Autodesk Inventor part; units mm, degrees
ref_plane "YZ Plane" through (0, 0, 0) normal (1, 0, 0) x (0, 1, 0)
ref_plane "XZ Plane" through (0, 0, 0) normal (0, 1, 0) x (-1, 0, 0)
ref_plane "XY Plane" through (0, 0, 0) normal (0, 0, 1) x (1, 0, 0)
sketch "スケッチ1" plane through (0, 0, 0) normal (0, 0, 1) x (1, 0, 0)
  line L0 (0, 0) -> (10, 0)
  line L1 (10, 0) -> (10, 30)
  line L2 (10, 30) -> (0, 30)
  line L3 (0, 30) -> (0, 0)
  dimension "d0" = 10
  dimension "d1" = 30
extrude "押し出し1" add sketch "スケッチ1" along normal blind 10
sketch "スケッチ2" plane through (0, 0, 10) normal (0, 0, 1) x (1, 0, 0)
  line L0 (10, 30) -> (0, 30)
  line L1 (10, 0) -> (10, 30)
  point P0 (0, 0)
  point P1 (5, 15)
  dimension "d4" = 15
  dimension "d5" = 5
hole "穴1" at (5, 15, 10) direction (0, 0, -1) diameter 4 end through all
sketch "スケッチ3" plane through (0, 0, 10) normal (0, 0, 1) x (1, 0, 0)
  point P0 (0, 0)
sketch "スケッチ4" plane through (0, 0, 10) normal (0, 0, 1) x (1, 0, 0)
  line L0 (10, 30) -> (0, 30)
  line L1 (10, 0) -> (10, 30)
  point P0 (0, 0)
  point P1 (5, 25)
  dimension "d13" = 5
  dimension "d14" = 5
hole "穴2" at (5, 25, 10) direction (0, 0, -1) diameter 2.459 end through all
sketch "スケッチ6" plane through (10, 0, 0) normal (1, 0, 0) x (0, 0, -1)
  line L0 (0, 0) -> (0, 30)
  line L1 (0, 30) -> (-10, 30)
  point P0 (-5, 15)
  dimension "d31" = 5
  dimension "d32" = 15
hole "穴4" at (10, 15, 5) direction (-1, 0, 0) diameter 2.459 end through all
sketch "スケッチ8" plane through (0, 0, 10) normal (0, 0, 1) x (1, 0, 0)
  line L0 (10, 0) -> (10, 30)
  line L1 (0, 0) -> (10, 0)
  point P0 (5, 5)
  dimension "d49" = 5
  dimension "d50" = 5
hole "穴6" at (5, 5, 10) direction (0, 0, -1) diameter 4 depth 10 tip angle 118 countersink diameter 5 countersink angle 90
properties part number "3SR05_振子固定パーツA"
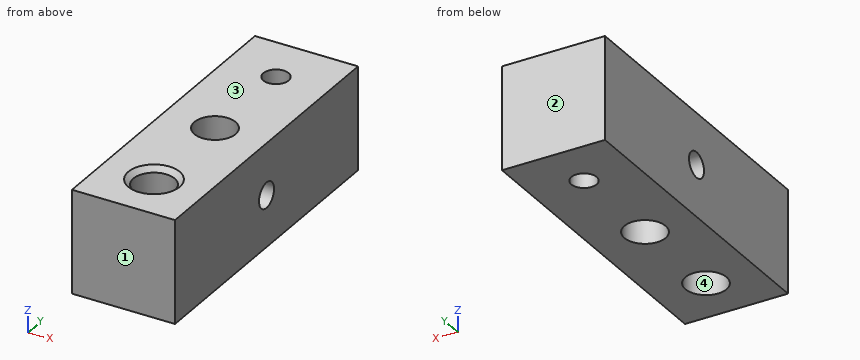
Here's how the part is built. I have some questions about the finished solid (model axes, mm). Face numbers are marked on the shaded views. Give positions to 0.01 mm unless a question says otherwise; leave off trailing zeros. Write each loop counter-clockwise with the first axis right and the second up, starting at its lowest first coordinate (ties: lowest second). Pieces come first, ordered by that corner, then holes. Notation, with made-up numbers: (69, -17) -> (86, -17) arc R19 cw to (86, 15) -> close; hole circle Ø6 at (20.25, 68.5). An arc over 180 degrees is marked (long way). Use one line per item in the form item = value.
1) We'd pull the mould along Y, two halves only. Please class the marked faces 1, 2, 3 and 4: +Y half, -Y half, draft (parallel to the pull), parting line (faces both ways), or undercut.
Verdict:
face_1 = -Y half
face_2 = +Y half
face_3 = draft
face_4 = undercut
2) If I drill on L1, parallel to Y at x = 8.8, z = 5; L2, parallel to Z at x = 9.3, y = 15; L3, parallel to X at y = 15, z = 3.5, over which ranges is the centre line in solid material (lowest first)? Write a range as [from, to].
Verdict:
L1 = [0, 13.77], [16.23, 30]
L2 = [0, 3.77], [6.23, 10]
L3 = [0, 3], [7, 10]
3) Suppose I cut it at D-D (y = 25). Please give me the cut outline in (x, z), and give its area (3 significant figures).
Verdict:
outline = (0, 0) -> (3.77, 0) -> (3.77, 10) -> (0, 10) -> close; (6.23, 0) -> (10, 0) -> (10, 10) -> (6.23, 10) -> close
area = 75.4 mm2
4) Suppose I cut it at C-C (z = 5.5). Please give me the cut outline in (x, y), and give its area (3 significant figures).
Verdict:
outline = (0, 0) -> (10, 0) -> (10, 13.88) -> (6.65, 13.88) arc R2 cw to (3.35, 13.88) -> (0, 13.88) -> close; (0, 16.12) -> (3.35, 16.12) arc R2 cw to (6.65, 16.12) -> (10, 16.12) -> (10, 30) -> (0, 30) -> close; hole circle Ø4 at (5, 5); hole circle Ø2.46 at (5, 25)
area = 256 mm2
5) Suppose I cut it at A-A (y = 15). Please give me the cut outline in (x, z).
Verdict:
outline = (0, 0) -> (3, 0) -> (3, 3.77) -> (0, 3.77) -> close; (0, 6.23) -> (3, 6.23) -> (3, 10) -> (0, 10) -> close; (7, 0) -> (10, 0) -> (10, 3.77) -> (7, 3.77) -> close; (7, 6.23) -> (10, 6.23) -> (10, 10) -> (7, 10) -> close
6) Suppose I cut it at B-B (x = 5). Please give me the cut outline in (y, z), and give its area (3 significant figures).
Verdict:
outline = (0, 0) -> (3, 0) -> (3, 9.5) -> (2.5, 10) -> (0, 10) -> close; (7, 0) -> (13, 0) -> (13, 10) -> (7.5, 10) -> (7, 9.5) -> close; (17, 0) -> (23.77, 0) -> (23.77, 10) -> (17, 10) -> close; (26.23, 0) -> (30, 0) -> (30, 10) -> (26.23, 10) -> close
area = 195 mm2
7) I'm going to push flat-ended pins straight in: pin 1 (3.5 mm diameter, centred on x = 5, y = 5, fed in from +Z); pin 2 (6 mm diameter, centred on x = 6, y = 15.5, fed in from -Z). Where does each tip first touch, or does it pass through?
Verdict:
pin_1 = through
pin_2 = 0
